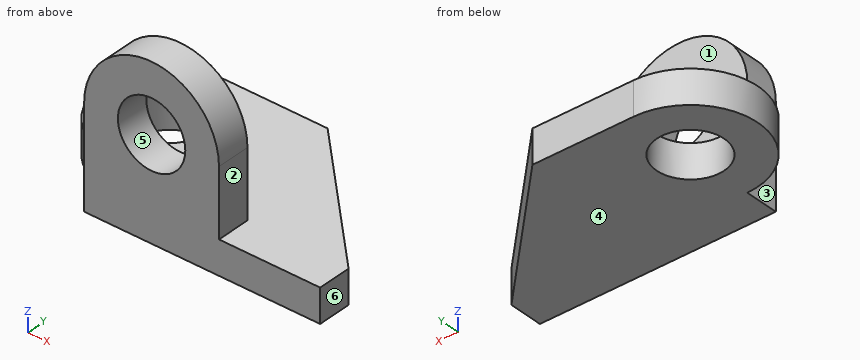
from build123d import *

# Parameters (mm, degrees)
SKETCH_1_R      = 5
EXTRUDE_1_DEPTH = 5
EXTRUDE_START   = -15
SKETCH_2_R      = 5
EXTRUDE_2_DEPTH = 5


with BuildPart() as part:
    # 草圖1 → 填料-伸長1 (new body)
    with BuildSketch(Plane.XY):
        with BuildLine():
            Line((0, 10), (15, 10))
            Line((15, 10), (35, -10))
            Line((35, -10), (35, -15))
            Line((35, -15), (0, -15))
            Line((0, -15), (0, -10))
            ThreePointArc((0, -10), (-10, 0), (0, 10))
        make_face()
        Circle(SKETCH_1_R, mode=Mode.SUBTRACT)
    extrude(amount=EXTRUDE_1_DEPTH)

    # 草圖2 → 填料-伸長2 (add)
    with BuildSketch(Plane(origin=(0, 0, 0), x_dir=(1, 0, 0), z_dir=(0, 1, 0)).offset(EXTRUDE_START)):
        with BuildLine():
            Line((0, -15), (0, -5))
            Line((0, -5), (20, -5))
            Line((20, -5), (20, -15))
            ThreePointArc((20, -15), (10, -25), (0, -15))
        make_face()
        with Locations((10, -15)):
            Circle(SKETCH_2_R, mode=Mode.SUBTRACT)
    extrude(amount=EXTRUDE_2_DEPTH)


solid = part.part
Model file for the job. Use its own axes, mm. Face numbers are marked on the shaded views. A direction names the side the tool comes from. Round coordinates to 2 decimals unless told otherwise and drop trailing zeros. Loops run counter-clockwise (first coordinate to the right, second up) from the corner with the lowest first, then second, coordinate; pieces in that order, holes last. Notation, with made-up numbers: (-16, 68) - (16, 68) arc R8 ccw to (16, 83) - close; hole circle Ø7 at (-22.5, 26). An arc over 180 degrees is marked (long way). Write each question's results on one line, items separated by ' | '.
(1) Pin check, flat tips, straight feed: pin 1 (6 mm diameter, centred on x = 0, y = 0, fed in from +Z); pin 2 (12.5 mm diameter, centred on x = 15.5, y = -1, fed in from +Z); pin 3 (4 mm diameter, centred on y = -12, z = 9.5, fed in from -X); pin 4 (5.5 mm diameter, centred on y = -13.5, z = 8, fed in from +X). Stop position of each tip, or through.
Answer below:
pin 1: passes through | pin 2: stops at z = 5 | pin 3: stops at x = 0 | pin 4: stops at x = 20
(2) Saw through at A-A, the plane y = 0. List the corners of the cut face in (x, z).
Answer below:
outline: (-10, 0) - (-5, 0) - (-5, 5) - (-10, 5) - close; (5, 0) - (25, 0) - (25, 5) - (5, 5) - close
(3) Saw through at B-B, the plane x = 10. List the corners of the cut face in (y, z).
Answer below:
outline: (-15, 0) - (10, 0) - (10, 5) - (-10, 5) - (-10, 10) - (-15, 10) - close; (-15, 20) - (-10, 20) - (-10, 25) - (-15, 25) - close
(4) Mould opens along X. For the marked faces 4, 5 and 6 say: released by +X, released by -X, zero draft, split by the parting line, or undercut.
Answer below:
face 4: zero draft | face 5: undercut | face 6: released by +X
(5) Saw through at D-D, the plane x = 27. List the corners of the cut face in (y, z).
Answer below:
outline: (-15, 0) - (-2, 0) - (-2, 5) - (-15, 5) - close
(6) Wall check: L1, parallel to Z at x = 10, y = -13.75; L2, parallel to Y at x = 14, z = 11.25; L3, parallel to Z at x = 18, y = 6.75. Give the ranges that are in metal, low to high.
Answer below:
L1: z = 0 to 10, 20 to 25 | L2: y = -15 to -10 | L3: z = 0 to 5
(7) Saw through at C-C, the plane z = 12.75. List the corners of the cut face in (x, y), then the cut area to 3 significant figures.
Answer below:
outline: (0, -15) - (5.53, -15) - (5.53, -10) - (0, -10) - close; (14.47, -15) - (20, -15) - (20, -10) - (14.47, -10) - close | area: 55.3 mm^2
(8) 3-axis set-ups, long thin cutter, end or side, ignore diameter. For the marked faces 1, 2 and 3: which of +Z, -Z, +X, -X, +Y, -Y reach the whole face in a straight line?
Answer below:
face 1: +Z, +X, -X, +Y | face 2: +Z, +X, +Y, -Y | face 3: +Z, -Z, -X, -Y
